For this review, take the finished solid that the model builds, in its own axes (mm). A direction names the side the tool comes from. Give positions to 0.01 mm unless a question says otherwise; leave off trailing zeros. Loops run counter-clockwise (first coordinate to the right, second up) from the corner with the lowest first, then second, coordinate; pieces in that order, holes last. Notation, with made-up numbers: (50.5, 73.5) -> (84.5, 73.5) arc R31 ccw to (84.5, 102.5) -> close; hole circle Ø7 at (80, 33.25). An arc over 180 degrees is marked (long way). One line per question, with ' | ' between items. Start each with the question number.
(1) Draft analysis for pull direction Z (two halves, no side actions). For faces 4 (the flat face through (85, 12, -94)), 5 (the flat face through (44, 0, -68)), 6 (the conical face through (4.01, 0.57, -131.13)), 7 (the flat face through (25, 13, -5)), state which applies: +Z half, -Z half, draft (parallel to the pull), parting line (faces both ways), or undercut.
(2) Consider section C-C (z = -112). Write out the cut boundary in (x, y).
(3) Consider section B-B (x = 52). Write out the cut boundary in (y, z), and give its area (3 significant figures).
(4) Tool access review of faces 1 (the flat face through (33, 12, -2)), 2 (the cylindrical face through (2, 17, -114)), 3 (the flat face through (46, 23, -68)): name each direction out of +Z, -Z, +X, -X, +Y, -Y from which nothing blocks a thin tool from reaching the whole face with its end or side.
(5) Wall thickness on probe 1 along Y at (x, z) = (4.5, -57.5); probe 2 along Y at (x, z) = (60, -3.1); probe 3 along X at (y, z) = (21, -9.5): over which ranges is each line inside the solid? List them lowest first.
(6) Consider section A-A (z = -28.5). Write out the cut boundary in (x, y).
(7) Insertion check: P1, Ø0.6, axis at x = 25, z = -134, coming from the -Y side; P2, Ø4, axis at x = 1.5, y = 11, coming from the -Z side; P3, Ø1, axis at y = 24, z = -81, coming from the +X side. Each pin has a flat end and moves straight along its axis. Give the tip position at first contact, or say it passes through.
(8) Consider section D-D (z = -71). Write out the cut boundary in (x, y).
from build123d import *

# Parameters (mm, degrees)
ESQUISSE1_W             = 90
ESQUISSE1_H             = 135
BOSS_EXTRU_1_DEPTH      = 25
CONG_1_R                = 10
CONG_2_R                = 10
CONG_3_R                = 10
CONG_4_R                = 10
CHANFREIN1_SIZE         = 2
CHANFREIN2_SIZE         = 2
ESQUISSE2_R             = 3
ESQUISSE2_W             = 8
ESQUISSE2_H             = 8
ESQUISSE2_W_2           = 15
ESQUISSE2_H_2           = 5
ENL_V_MAT_EXTRU_1_DEPTH = 5
ESQUISSE3_R             = 2
ESQUISSE3_W             = 75
ESQUISSE3_H             = 8
ENL_V_MAT_EXTRU_2_DEPTH = 5
ESQUISSE4_W             = 48
ESQUISSE4_H             = 72
ENL_V_MAT_EXTRU_3_DEPTH = 2
ENL_V_MAT_EXTRU_4_DEPTH = 2
ESQUISSE6_R             = 1.5
BOSS_EXTRU_2_DEPTH      = 2
ESQUISSE7_W             = 52
ESQUISSE7_H             = 10
ENL_V_MAT_EXTRU_5_DEPTH = 5


with BuildPart() as part:
    # Esquisse1 → Boss.-Extru.1 (new body)
    with BuildSketch(Plane(origin=(0, 0, 0), x_dir=(1, 0, 0), z_dir=(0, 1, 0))):
        with Locations((45, 67.5)):
            Rectangle(ESQUISSE1_W, ESQUISSE1_H)
    extrude(amount=BOSS_EXTRU_1_DEPTH)

    # Congé1
    cong_1_edges = [part.edges().sort_by_distance(p)[0] for p in [
        (90, 12.5, 0),
    ]]
    fillet(cong_1_edges, radius=CONG_1_R)

    # Congé2
    cong_2_edges = [part.edges().sort_by_distance(p)[0] for p in [
        (90, 12.5, -135),
    ]]
    fillet(cong_2_edges, radius=CONG_2_R)

    # Congé3
    cong_3_edges = [part.edges().sort_by_distance(p)[0] for p in [
        (0, 12.5, -135),
    ]]
    fillet(cong_3_edges, radius=CONG_3_R)

    # Congé4
    cong_4_edges = [part.edges().sort_by_distance(p)[0] for p in [
        (0, 12.5, 0),
    ]]
    fillet(cong_4_edges, radius=CONG_4_R)

    # Chanfrein1
    chanfrein1_edges = [part.edges().sort_by_distance(p)[0] for p in [
        (90, 25, -67.5),
        (87.071067812, 25, -2.928932188),
        (87.071067812, 25, -132.071067812),
        (45, 25, -135),
        (2.928932188, 25, -132.071067812),
        (45, 25, 0),
        (0, 25, -67.5),
        (2.928932188, 25, -2.928932188),
    ]]
    chamfer(chanfrein1_edges, length=CHANFREIN1_SIZE)

    # Chanfrein2
    chanfrein2_edges = [part.edges().sort_by_distance(p)[0] for p in [
        (90, 0, -67.5),
        (87.071067812, 0, -2.928932188),
        (87.071067812, 0, -132.071067812),
        (45, 0, -135),
        (2.928932188, 0, -132.071067812),
        (45, 0, 0),
        (0, 0, -67.5),
        (2.928932188, 0, -2.928932188),
    ]]
    chamfer(chanfrein2_edges, length=CHANFREIN2_SIZE)

    # Esquisse2 → Enlèv. mat.-Extru.1 (cut)
    with BuildSketch(Plane.XY):
        with Locations((60, 15)):
            Circle(ESQUISSE2_R)
        with Locations((46, 14)):
            Rectangle(ESQUISSE2_W, ESQUISSE2_H)
        with Locations((25.5, 12.5)):
            Rectangle(ESQUISSE2_W_2, ESQUISSE2_H_2)
    extrude(amount=-ENL_V_MAT_EXTRU_1_DEPTH, mode=Mode.SUBTRACT)

    # Esquisse3 → Enlèv. mat.-Extru.2 (cut)
    with BuildSketch(Plane.ZY):
        with Locations((-112, 17)):
            Circle(ESQUISSE3_R)
        with Locations((-100, 17)):
            Circle(ESQUISSE3_R)
        with Locations((-52.5, 13)):
            Rectangle(ESQUISSE3_W, ESQUISSE3_H)
    extrude(amount=-ENL_V_MAT_EXTRU_2_DEPTH, mode=Mode.SUBTRACT)

    # Esquisse4 → Enlèv. mat.-Extru.3 (cut)
    with BuildSketch(Plane(origin=(0, 25, 0), x_dir=(1, 0, 0), z_dir=(0, 1, 0))):
        with Locations((46, 67)):
            Rectangle(ESQUISSE4_W, ESQUISSE4_H)
    extrude(amount=-ENL_V_MAT_EXTRU_3_DEPTH, mode=Mode.SUBTRACT)

    # Esquisse5 → Enlèv. mat.-Extru.4 (cut)
    with BuildSketch(Plane(origin=(0, 0, -135), x_dir=(-1, 0, 0), z_dir=(0, 0, -1))):
        with BuildLine():
            Line((-30, 20), (-20, 20))
            ThreePointArc((-20, 20), (-15, 15), (-20, 10))
            Line((-20, 10), (-30, 10))
            ThreePointArc((-30, 10), (-35, 15), (-30, 20))
        make_face()
    extrude(amount=-ENL_V_MAT_EXTRU_4_DEPTH, mode=Mode.SUBTRACT)

    # Esquisse6 → Boss.-Extru.2 (add)
    with BuildSketch(Plane(origin=(0, 0, -133), x_dir=(-1, 0, 0), z_dir=(0, 0, -1))):
        with Locations(Location((-30, 15, 0), (0, 0, 180))):
            Circle(ESQUISSE6_R)
        with Locations(Location((-20, 15, 0), (0, 0, 180))):
            Circle(ESQUISSE6_R)
    extrude(amount=BOSS_EXTRU_2_DEPTH)

    # Esquisse7 → Enlèv. mat.-Extru.5 (cut)
    with BuildSketch(Plane(origin=(90, 0, 0), x_dir=(0, 0, -1), z_dir=(1, 0, 0))):
        with Locations((37, 12)):
            Rectangle(ESQUISSE7_W, ESQUISSE7_H)
        with Locations((94, 12)):
            Rectangle(ESQUISSE7_W, ESQUISSE7_H)
    extrude(amount=-ENL_V_MAT_EXTRU_5_DEPTH, mode=Mode.SUBTRACT)


solid = part.part
A:
1) face 4: undercut | face 5: draft | face 6: -Z half | face 7: +Z half
2) outline: (0, 2) -> (2, 0) -> (88, 0) -> (90, 2) -> (90, 7) -> (85, 7) -> (85, 17) -> (90, 17) -> (90, 23) -> (88, 25) -> (2, 25) -> (0, 23) -> (0, 19) -> (5, 19) -> (5, 15) -> (0, 15) -> close
3) outline: (0, -133) -> (2, -135) -> (23, -135) -> (25, -133) -> (25, -103) -> (23, -103) -> (23, -31) -> (25, -31) -> (25, -2) -> (23, 0) -> (2, 0) -> (0, -2) -> close | area: 3,220 mm^2
4) face 1: +Z | face 2: -X | face 3: +Y
5) probe 1: y = 0 to 9, 17 to 25 | probe 2: y = 0 to 12, 18 to 25 | probe 3: x = 0.01 to 89.99
6) outline: (0, 2) -> (2, 0) -> (88, 0) -> (90, 2) -> (90, 7) -> (85, 7) -> (85, 17) -> (90, 17) -> (90, 23) -> (88, 25) -> (2, 25) -> (0, 23) -> (0, 17) -> (5, 17) -> (5, 9) -> (0, 9) -> close
7) P1: stops at y = 0.7 | P2: stops at z = -132.6 | P3: stops at x = 89.5
8) outline: (0, 2) -> (2, 0) -> (88, 0) -> (90, 2) -> (90, 7) -> (85, 7) -> (85, 17) -> (90, 17) -> (90, 23) -> (88, 25) -> (70, 25) -> (70, 23) -> (22, 23) -> (22, 25) -> (2, 25) -> (0, 23) -> (0, 17) -> (5, 17) -> (5, 9) -> (0, 9) -> close
